from build123d import *

# Parameters (mm, degrees)
PAD_DEPTH    = 0.5
FILLET_R     = 0.24
PAD001_DEPTH = 3
FILLET001_R  = 0.5
SKETCH002_R  = 0.8
POCKET_DEPTH = 0.5
SKETCH003_R  = 0.7
PAD002_DEPTH = 0.5
SKETCH004_R  = 0.22
PAD003_DEPTH = 3


with BuildPart() as part:
    # Sketch → Pad (new body)
    with BuildSketch(Plane.XY):
        with BuildLine():
            Line((-3.2, 2.325), (3.2, 2.325))
            ThreePointArc((3.2, -2.325), (5.525, 0), (3.2, 2.325))
            Line((-3.2, -2.325), (3.2, -2.325))
            ThreePointArc((-3.2, 2.325), (-5.525, 0), (-3.2, -2.325))
        make_face()
    extrude(amount=PAD_DEPTH)

    # Fillet
    fillet_edges = [part.edges().sort_by_distance(p)[0] for p in [
        (0, -2.325, 0.5),
        (-5.525, 0, 0.5),
        (0, 2.325, 0.5),
        (5.525, 0, 0.5),
        (5.525, 0, 0),
        (0, -2.325, 0),
        (-5.525, 0, 0),
        (0, 2.325, 0),
    ]]
    fillet(fillet_edges, radius=FILLET_R)

    # Sketch001 (on DatumPlane) → Pad001 (join)
    with BuildSketch(Plane.XY.offset(0.5)):
        with BuildLine():
            Line((-3.2, 1.825), (3.2, 1.825))
            ThreePointArc((3.2, -1.825), (5.025, 0), (3.2, 1.825))
            Line((-3.2, -1.825), (3.2, -1.825))
            ThreePointArc((-3.2, 1.825), (-5.025, 0), (-3.2, -1.825))
        make_face()
    extrude(amount=PAD001_DEPTH)

    # Fillet001
    fillet001_edges = [part.edges().sort_by_distance(p)[0] for p in [
        (0, -1.825, 3.5),
        (-5.025, 0, 3.5),
        (0, 1.825, 3.5),
        (5.025, 0, 3.5),
    ]]
    fillet(fillet001_edges, radius=FILLET001_R)

    # Sketch002 (on DatumPlane) → Pocket (cut)
    with BuildSketch(Plane.XY.offset(0.5)):
        with Locations((-2.44, 0)):
            Circle(SKETCH002_R)
        with Locations((2.44, 0)):
            Circle(SKETCH002_R)
    extrude(amount=-POCKET_DEPTH, mode=Mode.SUBTRACT)

    # Sketch003 (on DatumPlane) → Pad002 (join)
    with BuildSketch(Plane.XY.offset(0.5)):
        with Locations((2.44, 0)):
            Circle(SKETCH003_R)
        with Locations((-2.44, 0)):
            Circle(SKETCH003_R)
    extrude(amount=-PAD002_DEPTH)

    # Sketch004 → Pad003 (join)
    with BuildSketch(Plane.XY):
        with Locations((2.44, 0)):
            Circle(SKETCH004_R)
        with Locations((-2.44, 0)):
            Circle(SKETCH004_R)
    extrude(amount=-PAD003_DEPTH)


solid = part.part
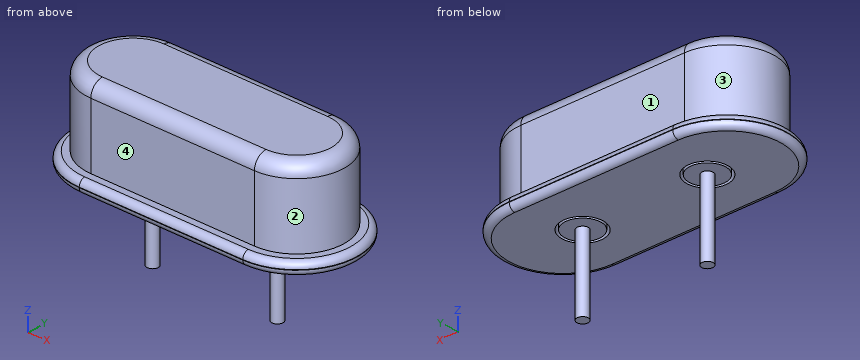
Check sheet for the modelled part. Datum: model origin and axes. Units: mm. Face numbers are marked on the shaded views. A direction names the side the tool comes from. Round coordinates to 2 decimals unless told otherwise and drop trailing zeros. Loops run counter-clockwise (first coordinate to the right, second up) from the corner with the lowest first, then second, coordinate; pieces in that order, holes last. Notation, with made-up numbers: M 79.25,-17 L 119.25,-17 A28 ccw 119.25,12 Z; hole C -4.5,-10.75 d7. An arc over 180 degrees is marked long. One line per question, with ' | ' between items. Start each with the question number.
Item 1: Set-up check for the marked faces 1, 2, 3 and 4: record each of +Z, -Z, +X, -X, +Y, -Y from which the full face is reachable in a straight line by a thin tool's end or side.
Item 2: Gauge pin test, flat ends, axial feed: pin 1 Ø2 at (x, z) = (-2, -2) entering from +Y; pin 2 Ø1.3 at (x, y) = (0.5, -0.5) entering from -Z; pin 3 Ø1 at (y, z) = (-0.5, 2) entering from +X (3 decimals). Record the tip position at first contact, or that the pin passes through.
Item 3: Scan lines: probe 1 along Z at (x, y) = (-0.25, -0.85); probe 2 along Y at (x, z) = (2.5, 1) (3 decimals); probe 3 along Z at (x, y) = (3.5, 2). Record each from-to range of solid material in increasing order.
Item 4: Section check A-A (x = -0.5). Record the boundary of the cut face in (y, z) (3 decimals), and give its area (3 significant figures).
Item 5: Section check B-B (z = 1.25). Record the boundary of the cut face in (x, y) (3 decimals), and give its area (3 significant figures).
Item 6: Section check C-C (x = 2.44). Record the boundary of the cut face in (y, z) (3 decimals).
Worked out:
1) face 1: +Z, +X, -X, +Y | face 2: +Z, +X | face 3: +Z, -X | face 4: +Z, +X, -X, -Y
2) pin 1: y = 0.22 | pin 2: z = 0 | pin 3: x = 5.025
3) probe 1: 0 to 3.5 | probe 2: -1.825 to 1.825 | probe 3: 0 to 0.5
4) outline: M -2.325,0.24 A0.24 ccw -2.085,0 L 2.085,0 A0.24 ccw 2.325,0.24 L 2.325,0.26 A0.24 ccw 2.085,0.5 L 1.825,0.5 L 1.825,3 A0.5 ccw 1.325,3.5 L -1.325,3.5 A0.5 ccw -1.825,3 L -1.825,0.5 L -2.085,0.5 A0.24 ccw -2.325,0.26 Z | area: 13.1 mm^2
5) outline: M -3.2,-1.825 L 3.2,-1.825 A1.825 ccw 3.2,1.825 L -3.2,1.825 A1.825 ccw Z | area: 33.8 mm^2
6) outline: M -2.325,0.24 A0.24 ccw -2.085,0 L -0.8,0 L -0.8,0.5 L -0.7,0.5 L -0.7,0 L -0.22,0 L -0.22,-3 L 0.22,-3 L 0.22,0 L 0.7,0 L 0.7,0.5 L 0.8,0.5 L 0.8,0 L 2.085,0 A0.24 ccw 2.325,0.24 L 2.325,0.26 A0.24 ccw 2.085,0.5 L 1.825,0.5 L 1.825,3 A0.5 ccw 1.325,3.5 L -1.325,3.5 A0.5 ccw -1.825,3 L -1.825,0.5 L -2.085,0.5 A0.24 ccw -2.325,0.26 Z
